Geometry check sheet. Reference: the model listing, model coordinates, mm. A direction names the side the tool comes from. Give positions to 0.01 mm unless a question says otherwise; leave off trailing zeros. Write each loop counter-clockwise with the first axis right and the second up, starting at its lowest first coordinate (ties: lowest second). Pieces come first, ordered by that corner, then holes. Notation, with made-up numbers: (59.25, 52.5) -> (113.25, 52.5) arc R25 ccw to (113.25, 75.5) -> close; hole circle Ø4 at (-25, 9). An arc over 180 degrees is marked (long way). Write item = value, one per line. Start each with the question number.
1. Cross-section at C-C, the plane y = -4. Record the cut outline in (x, z), plus the area to 3 significant figures.
2. Mould release check, pull along Z, two halves, no side actions. Record for faces 1 (the flat face through (-3, -6.9, -38.1)), 2 (the flat face through (-19.05, -13, 48)), 3 (the flat face through (-4, -18, 63.5)), 4 (the flat face through (4, -18, -63.5)): pulls with the +Z half, pulls with the -Z half, needs draft (parallel to the pull), parting line crosses it, or undercut.
3. Cross-section at D-D, the plane x = -5. State how many separate pieces and enclosed holes the cut face has, plus the area to 3 significant figures.
4. Thickness scan on line 1 along X through (y, z) = (-22.5, -1); line 2 along Z through (x, y) = (12, -3.5); line 3 along Z through (x, y) = (-10.5, -16.75). Record the ranges inside material, lowest first.
5. Depth check by flat-ended pin: P1, Ø7.5, axis at y = -18.5, z = 50.5, coming from the -X side; P2, Ø11.5, axis at x = 0, y = -12.7, coming from the +Z side; P3, Ø2, axis at y = -18, z = 17.5, coming from the +X side; P4, Ø12, axis at y = -20.5, z = 8, coming from the -X side. Enter the tip coordinate at first touch or a pass-through.
6. Cross-section at A-A, the plane x = 27. Record the cut outline in (y, z), plus the area to 3 significant figures.
7. Set-up check for faces 5 (the flat face through (-3, -6.9, 57.15)), 6 (the flat face through (19.05, -13, -48)), 7 (the flat face through (0, -25.4, 33)), 8 (the flat face through (19.05, -13, 48)), 9 (the flat face through (-19.05, -13, -48)): record each of +Z, -Z, +X, -X, +Y, -Y from which the full face is reachable in a straight line by a thin tool's end or side.
8. Cross-section at B-B, the plane z = -43. Record the cut outline in (x, y), plus the area to 3 significant figures.
```python
from build123d import *

# Parameters (mm, degrees)
F0_R     = 31.75
F0_W     = 6.35
F0_H     = 6.35
F0_H_2   = 6.514672
F1_DEPTH = 25.4
F3_DEPTH = 102.108
F4_DEPTH = 65.278


with BuildPart() as f1:
    # F0 (on Front) → F1 (new body)
    with BuildSketch(Plane.XZ):
        with BuildLine():
            ThreePointArc((19.05, -32.995568), (32.995568, -19.05), (38.1, 0))
            ThreePointArc((38.1, 0), (32.995568, 19.05), (19.05, 32.995568))
            ThreePointArc((19.05, 32.995568), (9.861006, 36.801774), (0, 38.1))
            ThreePointArc((0, 38.1), (-9.861006, 36.801774), (-19.05, 32.995568))
            ThreePointArc((-19.05, 32.995568), (-38.1, 0), (-19.05, -32.995568))
            ThreePointArc((-19.05, -32.995568), (-9.861006, -36.801774), (0, -38.1))
            ThreePointArc((0, -38.1), (9.861006, -36.801774), (19.05, -32.995568))
        make_face()
        Circle(F0_R, mode=Mode.SUBTRACT)
        with BuildLine():
            ThreePointArc((0, 38.1), (9.861006, 36.801774), (19.05, 32.995568))
            Line((19.05, 32.995568), (19.05, 38.1))
            Line((19.05, 38.1), (12.7, 38.1))
            Line((12.7, 38.1), (0, 38.1))
        make_face()
        with BuildLine():
            Line((19.05, -38.1), (19.05, -32.995568))
            ThreePointArc((19.05, -32.995568), (9.861006, -36.801774), (0, -38.1))
            Line((0, -38.1), (12.7, -38.1))
            Line((12.7, -38.1), (19.05, -38.1))
        make_face()
        with BuildLine():
            ThreePointArc((-19.05, 32.995568), (-9.861006, 36.801774), (0, 38.1))
            Line((0, 38.1), (-12.7, 38.1))
            Line((-12.7, 38.1), (-19.05, 38.1))
            Line((-19.05, 38.1), (-19.05, 32.995568))
        make_face()
        with Locations((15.875, 41.275)):
            Rectangle(F0_W, F0_H)
        with BuildLine():
            Line((-12.7, -38.1), (0, -38.1))
            ThreePointArc((0, -38.1), (-9.861006, -36.801774), (-19.05, -32.995568))
            Line((-19.05, -32.995568), (-19.05, -38.1))
            Line((-19.05, -38.1), (-12.7, -38.1))
        make_face()
        with Locations((15.875, -41.357336)):
            Rectangle(F0_W, F0_H_2)
        with Locations((-15.875, 41.275)):
            Rectangle(F0_W, F0_H)
        Polygon((12.7, 44.45), (19.05, 44.45), (19.05, 63.5), (-19.05, 63.5), (-19.05, 44.45), (-12.7, 44.45), (-12.7, 57.15), (12.7, 57.15), align=None)
        with Locations((-15.875, -41.275)):
            Rectangle(F0_W, F0_H)
        Polygon((19.05, -63.5), (19.05, -44.614672), (12.7, -44.614672), (12.7, -57.314672), (-12.7, -57.15), (-12.7, -44.45), (-19.05, -44.45), (-19.05, -63.5), align=None)
    extrude(amount=F1_DEPTH)

    # F2 (on Top) → F3 (cut)
    with BuildSketch(Plane.XY):
        with BuildLine():
            ThreePointArc((0, -6.35), (-4.490128, -17.190128), (6.35, -12.7))
            ThreePointArc((6.35, -12.7), (4.490128, -8.209872), (0, -6.35))
        make_face()
    extrude(amount=-F3_DEPTH, mode=Mode.SUBTRACT)

    # F2 (on Top) → F4 (cut)
    with BuildSketch(Plane.XY):
        with BuildLine():
            ThreePointArc((0, -6.35), (-4.490128, -17.190128), (6.35, -12.7))
            ThreePointArc((6.35, -12.7), (4.490128, -8.209872), (0, -6.35))
        make_face()
    extrude(amount=F4_DEPTH, mode=Mode.SUBTRACT)


solid = f1.part
```
Answers:
q1.outline = (-19.05, -63.5) -> (19.05, -63.5) -> (19.05, -33) arc R38.1 ccw to (19.05, 33) -> (19.05, 63.5) -> (-19.05, 63.5) -> (-19.05, 33) arc R38.1 ccw to (-19.05, -33) -> close; hole circle Ø63.5 at (0, 0); hole (-12.7, -57.15) -> (12.7, -57.31) -> (12.7, -38.1) -> (-12.7, -38.1) -> close; hole (-12.7, 38.1) -> (12.7, 38.1) -> (12.7, 57.15) -> (-12.7, 57.15) -> close
q1.area = 2,490 mm^2
q2.face_1 = undercut
q2.face_2 = needs draft
q2.face_3 = pulls with the +Z half
q2.face_4 = pulls with the -Z half
q3.separate_pieces = 8
q3.enclosed_holes = 0
q3.area = 459 mm^2
q4.line_1 = -38.09 to -31.73, 31.73 to 38.09
q4.line_2 = -63.5 to -57.31, -38.1 to -29.39, 29.39 to 38.1, 57.15 to 63.5
q4.line_3 = -63.5 to -57.16, -38.1 to -29.96, 29.96 to 38.1, 57.15 to 63.5
q5.P1 = -19.05
q5.P2 = through
q5.P3 = 34.34
q5.P4 = -38.05
q6.outline = (-25.4, -26.88) -> (0, -26.88) -> (0, -16.71) -> (-25.4, -16.71) -> close; (-25.4, 16.71) -> (0, 16.71) -> (0, 26.88) -> (-25.4, 26.88) -> close
q6.area = 517 mm^2
q7.face_5 = +Y, -Y
q7.face_6 = -Z, +X, +Y, -Y
q7.face_7 = +Z, -Z, +X, -X, -Y
q7.face_8 = +Z, +X, +Y, -Y
q7.face_9 = -Z, -X, +Y, -Y
q8.outline = (-19.05, -25.4) -> (-12.7, -25.4) -> (-12.7, 0) -> (-19.05, 0) -> close; (12.7, -25.4) -> (19.05, -25.4) -> (19.05, 0) -> (12.7, 0) -> close
q8.area = 323 mm^2
